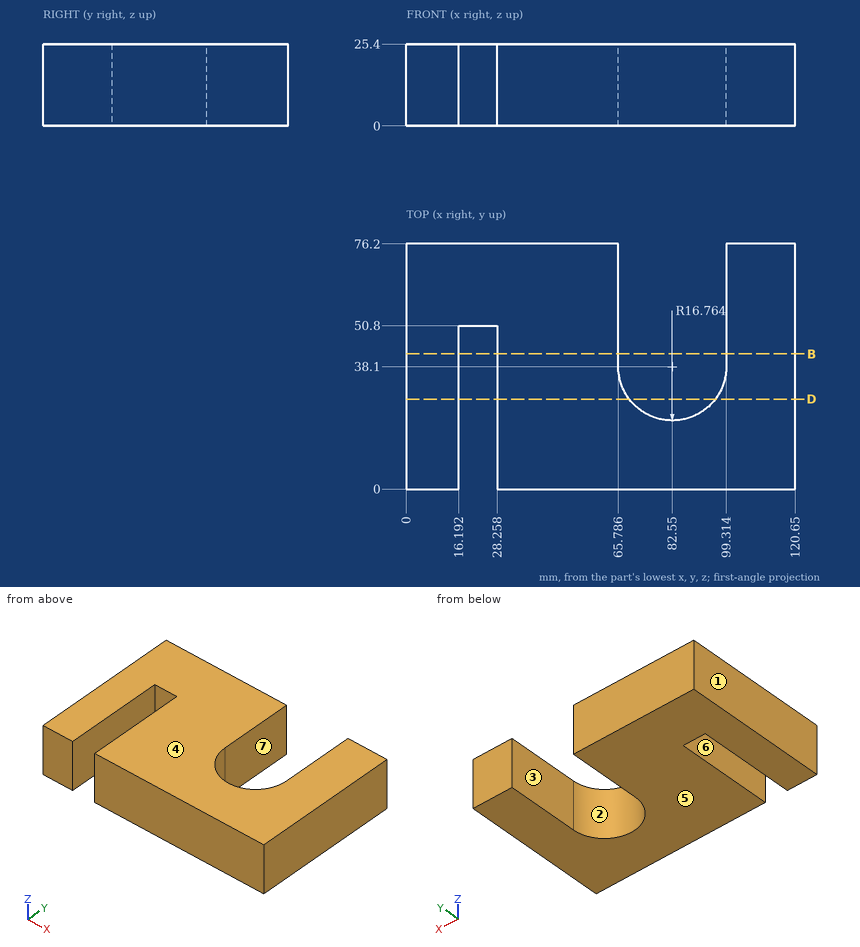
For this review, use the dimensioned drawing (mm, ordinates from the lowest corner) and the shaded views. A direction names the side the tool comes from. Coordinates: 2 decimals unless noted, no trailing zeros. Loops run counter-clockwise (first coordinate to the right, second up) from the corner with the lowest first, then second, coordinate; pieces in that order, holes last. Notation, with made-up numbers: (5, 50.5) -> (59, 50.5) arc R26 cw to (59, 65.5) -> close; hole circle Ø9 at (38, 86.25). An arc over 180 degrees is marked (long way). Use a Markdown table: item, result. Add a question column.
Item 1: We need section D-D, the plane y = 28. Write out the cut boundary in (x, z).
Item 2: Wall thickness on L1, parallel to X at y = 37.5, z = 20.75; L2, parallel to X at y = 12, z = 11; L3, parallel to X at y = 34.5, z = 19: over which ranges is each line inside the solid? List them lowest first. Write a range as from..to.
Item 3: We need section B-B, the plane y = 42. Count the separate pieces of the cut face and the enclosed holes in it, and give its area (3 significant figures).
Item 4: Clearance check with flat-ended pins moving along their axes: P1, Ø6, axis at x = 106, y = 28.5, coming from the -Z side; P2, Ø6, axis at x = 23.5, z = 17.5, coming from the -Y side. State where each tip first meets the part, or that it passes through.
Item 5: The part is to be moulded in two halves that separate along X. For the marked faces 1, 2, 3 and 4, say which applies: +X half, -X half, draft (parallel to the pull), parting line (faces both ways), or undercut.
Item 6: Machinability: for the marked faces 5, 6 and 7, which of the approach directions +Z, -Z, +X, -X, +Y, -Y give a long, thin tool a straight path to every point of the face, cutting with its end or side? Answer none if there is none.
Numbers:
| question | item | result |
|---|---|---|
| 1 | outline | (0, 0) -> (16.19, 0) -> (16.19, 25.4) -> (0, 25.4) -> close; (28.26, 0) -> (69.17, 0) -> (69.17, 25.4) -> (28.26, 25.4) -> close; (95.93, 0) -> (120.65, 0) -> (120.65, 25.4) -> (95.93, 25.4) -> close |
| 2 | L1 | x = 0..16.19, 28.26..65.8, 99.3..120.65 |
| 2 | L2 | x = 0..16.19, 28.26..120.65 |
| 2 | L3 | x = 0..16.19, 28.26..66.18, 98.92..120.65 |
| 3 | separate pieces | 3 |
| 3 | enclosed holes | 0 |
| 3 | area | 1,910 mm^2 |
| 4 | P1 | stops at z = 0 |
| 4 | P2 | stops at y = 50.8 |
| 5 | face 1 | -X half |
| 5 | face 2 | undercut |
| 5 | face 3 | undercut |
| 5 | face 4 | draft |
| 6 | face 5 | -Z, +X, -X, +Y, -Y |
| 6 | face 6 | +Z, -Z, -Y |
| 6 | face 7 | +Z, -Z, +Y |
